Autodesk Inventor part; units mm, degrees
ref_plane "YZ Plane" through (0, 0, 0) normal (1, 0, 0) x (0, 1, 0)
ref_plane "XZ Plane" through (0, 0, 0) normal (0, 1, 0) x (-1, 0, 0)
ref_plane "XY Plane" through (0, 0, 0) normal (0, 0, 1) x (1, 0, 0)
sketch "スケッチ1" plane through (0, 0, 0) normal (0, 0, 1) x (1, 0, 0)
  circle A0 centre (-35, 0) radius 1.6
  circle A1 centre (35, 0) radius 1.6
  circle A2 centre (-87.5, 39.5) radius 1.6
  circle A3 centre (87.5, 39.5) radius 1.6
  arc A4 (-85.3659, 44.0217) -> (-90.4756, 35.4818) centre (-87.5, 39.5) ccw
  arc A5 (-37.678, -3.6164) -> (-35, -4.5) centre (-35, 0) ccw
  arc A6 (35, -4.5) -> (37.678, -3.6164) centre (35, 0) ccw
  arc A7 (90.4756, 35.4818) -> (85.3659, 44.0217) centre (87.5, 39.5) ccw
  arc A8 (-85.3659, 44.0217) -> (85.3659, 44.0217) centre (0, 224.8881) ccw
  line L0 (-90.4756, 35.4818) -> (-37.678, -3.6164)
  line L1 (-35, -4.5) -> (35, -4.5)
  line L2 (37.678, -3.6164) -> (90.4756, 35.4818)
  point P0 (0, 0)
  dimension "d0" = 3.2
  dimension "d1" = 3.2
  dimension "d2" = 70
  dimension "d3" = 35
  dimension "d4" = 3.2
  dimension "d5" = 3.2
  dimension "d6" = 39.5
  dimension "d7" = 175
  dimension "d8" = 87.5
  dimension "d9" = 5
  dimension "d10" = 4.5
  dimension "d11" = 4.5
  dimension "d12" = 5
  dimension "d13" = 200
extrude "押し出し1" add sketch "スケッチ1" along normal blind 3
properties part number "ハンド_下側板" material "アルミニウム 6061"
CAD build for the part. Positions are in the model's coordinates, mm. Round coordinates to 2 decimals unless told otherwise and drop trailing zeros. Write each loop counter-clockwise with the first axis right and the second up, starting at its lowest first coordinate (ties: lowest second). Pieces come first, ordered by that corner, then holes. Notation, with made-up numbers: (-26.5, 56.5) -> (0.5, 56.5) arc R34 cw to (0.5, 86.5) -> close; hole circle Ø4 at (-18.75, -28). An arc over 180 degrees is marked (long way). Answer in a Markdown table with one row per item. Add a question column.
Item 1: Saw through at A-A, the plane y = 33.5. Write the cut outline in (x, z).
Item 2: Drill centre lines: line 1 (X direction, y = 1, z = 1.75); line 2 (Y direction, x = 35, z = 1.45); line 3 (Y direction, x = 34, z = 0.8). Where is each one in solid material? Low to high. Write a range as from..to.
Item 3: Saw through at D-D, the plane x = -63.5. Write the cut outline in (y, z), then the cut area to 3 significant figures.
Item 4: Saw through at B-B, the plane z = 1.4. Write the cut outline in (x, y), then the cut area to 3 significant figures.
Item 5: Saw through at C-C, the plane x = 87.5. Write the cut outline in (y, z).
Item 6: Mould opens along Y. For faces 1 (the face through (-88.77, 40.47, 1.48)), 2 (the face through (-91.84, 41.98, 1.48)), 3 (the face through (63.71, 15.66, 1.48)), 4 (the face through (-36.18, -1.08, 1.48)) say: pulls with the +Y half, pulls with the -Y half, needs draft (parallel to the pull), parting line crosses it, or undercut.
Findings below:
| question | item | result |
|---|---|---|
| 1 | outline | (-87.8, 0) -> (-58.06, 0) -> (-58.06, 3) -> (-87.8, 3) -> close; (58.06, 0) -> (87.8, 0) -> (87.8, 3) -> (58.06, 3) -> close |
| 2 | line 1 | x = -43.91..-36.25, -33.75..33.75, 36.25..43.91 |
| 2 | line 2 | y = -4.5..-1.6, 1.6..27.97 |
| 2 | line 3 | y = -4.5..-1.25, 1.25..27.8 |
| 3 | outline | (15.51, 0) -> (35.24, 0) -> (35.24, 3) -> (15.51, 3) -> close |
| 3 | area | 59.2 mm^2 |
| 4 | outline | (-90.48, 35.48) -> (-37.68, -3.62) arc R4.5 ccw to (-35, -4.5) -> (35, -4.5) arc R4.5 ccw to (37.68, -3.62) -> (90.48, 35.48) arc R5 ccw to (85.37, 44.02) arc R200 cw to (-85.37, 44.02) arc R5 ccw to start; hole circle Ø3.2 at (-87.5, 39.5); hole circle Ø3.2 at (-35, 0); hole circle Ø3.2 at (35, 0); hole circle Ø3.2 at (87.5, 39.5) |
| 4 | area | 4,410 mm^2 |
| 5 | outline | (33.28, 0) -> (37.9, 0) -> (37.9, 3) -> (33.28, 3) -> close; (41.1, 0) -> (44.5, 0) -> (44.5, 3) -> (41.1, 3) -> close |
| 6 | face 1 | undercut |
| 6 | face 2 | parting line crosses it |
| 6 | face 3 | pulls with the -Y half |
| 6 | face 4 | undercut |
